Work out the finished part from the listing and answer in its coordinate system (mm). Face numbers are marked on the shaded views. A direction names the side the tool comes from. Coordinates: 2 decimals unless noted, no trailing zeros. Write each loop counter-clockwise with the first axis right and the second up, starting at its lowest first coordinate (ties: lowest second). Pieces come first, ordered by that corner, then holes. Notation, with made-up numbers: M -10.5,-16.75 L -3.5,-16.75 A30 ccw -3.5,13.25 Z; hole C -1.5,-22 d1. An arc over 180 degrees is marked long. Use CSV: the item, a comma, the result in double quotes.
from build123d import *

# Parameters (mm, degrees)
SKETCH1_R           = 11.7
SKETCH1_R_2         = 9.7
BOSS_EXTRUDE1_DEPTH = 5
BOSS_EXTRUDE2_START = 1
SKETCH2_R           = 11.7
BOSS_EXTRUDE2_DEPTH = 1
SKETCH3_W           = 8
SKETCH3_H           = 2
CUT_EXTRUDE1_DEPTH  = 7


with BuildPart() as part:
    # Sketch1 → Boss-Extrude1 (new body)
    with BuildSketch(Plane(origin=(0, 0, 0), x_dir=(1, 0, 0), z_dir=(0, 1, 0))):
        with Locations(Location((0, 0, 0), (0, 0, 270))):
            Circle(SKETCH1_R)
        with Locations(Location((0, 0, 0), (0, 0, 270))):
            Circle(SKETCH1_R_2, mode=Mode.SUBTRACT)
    extrude(amount=BOSS_EXTRUDE1_DEPTH)

    # Sketch2 → Boss-Extrude2 (add)
    with BuildSketch(Plane.XZ.offset(BOSS_EXTRUDE2_START)):
        with Locations(Location((0, 0, 0), (0, 0, 270))):
            Circle(SKETCH2_R)
    extrude(amount=-BOSS_EXTRUDE2_DEPTH)

    # Sketch3 → Cut-Extrude1 (cut)
    with BuildSketch(Plane.XZ.offset(1)):
        Rectangle(SKETCH3_W, SKETCH3_H)
    extrude(amount=-CUT_EXTRUDE1_DEPTH, mode=Mode.SUBTRACT)


solid = part.part
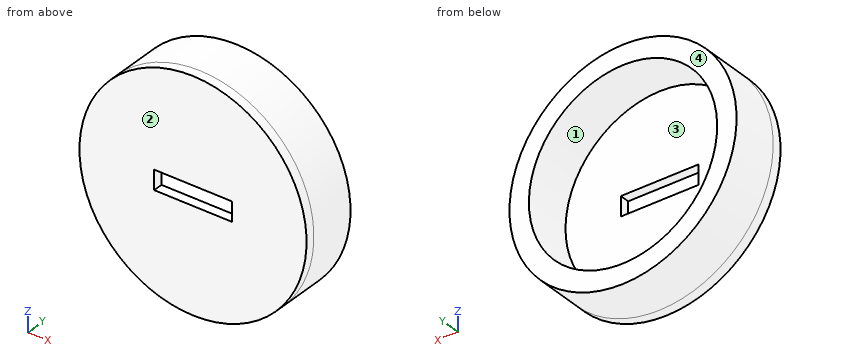
Item 1: Given pin 1 (2 mm diameter, centred on x = 4.5, z = -0.5, fed in from +Y); pin 2 (1.5 mm diameter, centred on x = -5.5, y = 4, fed in from -Z); pin 3 (2 mm diameter, centred on y = -0.5, z = -5.5, fed in from +X), each flat-ended and moving along its own axis, determine where each tip first touches the part or whether it passes through.
Answer:
pin 1,"stops at y = 0"
pin 2,"stops at z = -10.69"
pin 3,"stops at x = 10.8"
Item 2: A tool of negligible diameter and unlimited length cuts with its end or side. For the marked faces 3 and 4, from which of +Z, -Z, +X, -X, +Y, -Y can it reach the whole face along a straight path? Write none if from no direction.
Answer:
face 3,"+Y"
face 4,"+Z, -Z, +X, -X, +Y"
Item 3: The part is cut by section A-A (z = 0). Write down the section's boundary in (x, y), then the cut area to 3 significant figures.
Answer:
outline,"M -11.7,-1 L -4,-1 L -4,0 L -9.7,0 L -9.7,5 L -11.7,5 Z; M 4,-1 L 11.7,-1 L 11.7,5 L 9.7,5 L 9.7,0 L 4,0 Z"
area,"35.4 mm2"
Item 4: The part is cut by section B-B (x = 0). Write down the section's boundary in (y, z).
Answer:
outline,"M -1,-11.7 L 5,-11.7 L 5,-9.7 L 0,-9.7 L 0,-1 L -1,-1 Z; M -1,1 L 0,1 L 0,9.7 L 5,9.7 L 5,11.7 L -1,11.7 Z"
Item 5: Consider probe 1 along X at (y, z) = (2.6, 0); probe 2 along Y at (x, z) = (2.75, -6.75); probe 3 along Z at (x, y) = (4.75, 0.7). Determine where each line is inside the solid, lowest interval first.
Answer:
probe 1,"x = -11.7 to -9.7, 9.7 to 11.7"
probe 2,"y = -1 to 0"
probe 3,"z = -10.69 to -8.46, 8.46 to 10.69"
Item 6: The part is cut by section D-D (z = -5.25). Write down the section's boundary in (x, y), then the cut area to 3 significant figures.
Answer:
outline,"M -10.46,-1 L 10.46,-1 L 10.46,5 L 8.16,5 L 8.16,0 L -8.16,0 L -8.16,5 L -10.46,5 Z"
area,"43.9 mm2"
Item 7: For a pull along Z with two mould halves and no side action, classify the marked faces 1 and 2 as released by +Z, released by -Z, zero draft, split by the parting line, or undercut.
Answer:
face 1,"undercut"
face 2,"zero draft"
Item 8: The part is cut by section C-C (y = 1.95). Write down the section's boundary in (x, z).
Answer:
outline,"C 0,0 d23.4; hole C 0,0 d19.4"
